Geometry: final body of the model. Coordinates: model frame, mm. Face numbers are marked on the shaded views. A direction names the side the tool comes from. Round coordinates to 2 decimals unless told otherwise and drop trailing zeros. Loops run counter-clockwise (first coordinate to the right, second up) from the corner with the lowest first, then second, coordinate; pieces in that order, holes last. Notation, with made-up numbers: (-34.75, 10) - (-22.75, 10) arc R18 cw to (-22.75, 41) - close; hole circle Ø2 at (59.25, 53.25). An arc over 180 degrees is marked (long way). Return JSON: item names as keys, results as strings. Group by question number.
1. Material intervals for probe 1 along Z at (x, y) = (6.5, 2.5); probe 2 along Z at (x, y) = (8, 4.5); probe 3 along Y at (x, z) = (0.75, 0.95), sorted ascending.
2. Section C-C on z = 0.55. Return loops of the section in (x, y), and give its area (3 significant figures).
3. Section D-D on x = 7.5. Return loops of the section in (y, z).
4. First-contact query: pin 1 Ø0.8 at (x, z) = (4, 0.5) entering from +Y; pin 2 Ø0.8 at (x, z) = (3.5, 0.5) entering from -Y. Flat tips, straight axial feed; report the tip coordinate or a pass-through.
5. Section B-B on x = 5.75. Return loops of the section in (y, z), and give its area (3 significant figures).
6. Set-up query: the marked faces 1, 2 and 3. Return all of +Z, -Z, +X, -X, +Y, -Y with unobstructed straight access to the full face (end or side cutting, diameter ignored); none if empty.
7. Section A-A on y = 0.75. Return loops of the section in (x, z).
from build123d import *

# Parameters (mm, degrees)
SKIZZE1_W                       = 6.912
SKIZZE1_H                       = 3.888
AUFSATZ_LINEAR_AUSTRAGEN1_DEPTH = 1
SKIZZE2_W                       = 10.912
SKIZZE2_H                       = 7.888
AUFSATZ_LINEAR_AUSTRAGEN2_DEPTH = 1
AUFSATZ_LINEAR_AUSTRAGEN3_DEPTH = 0.48
SCHNITT_LINEAR_AUSTRAGEN1_DEPTH = 40.48
SKIZZE7_R                       = 0.1
SCHNITT_LINEAR_AUSTRAGEN2_DEPTH = 0.1
SKIZZE8_R                       = 0.1
SCHNITT_LINEAR_AUSTRAGEN3_DEPTH = 0.1


with BuildPart() as part:
    # Skizze1 → Aufsatz-Linear austragen1 (new body)
    with BuildSketch(Plane.XY):
        with Locations((3.456, 1.944)):
            Rectangle(SKIZZE1_W, SKIZZE1_H)
    extrude(amount=AUFSATZ_LINEAR_AUSTRAGEN1_DEPTH)

    # Skizze2 → Aufsatz-Linear austragen2 (add)
    with BuildSketch(Plane.XY.offset(1)):
        with Locations((3.456, 1.944)):
            Rectangle(SKIZZE2_W, SKIZZE2_H)
    extrude(amount=AUFSATZ_LINEAR_AUSTRAGEN2_DEPTH)

    # Skizze3 → Aufsatz-Linear austragen3 (add)
    with BuildSketch(Plane(origin=(0, 0, 0), x_dir=(-1, 0, 0), z_dir=(0, 0, -1))):
        Polygon((-3.956, 1.944), (-3.456, 2.444), (-2.961061255, 1.949061255), (-3.461061255, 1.449061255), align=None)
    extrude(amount=AUFSATZ_LINEAR_AUSTRAGEN3_DEPTH)

    # Skizze6 → Schnitt-Linear austragen1 (cut)
    with BuildSketch(Plane(origin=(1.006, -1.006, 0), x_dir=(0, 0, -1), z_dir=(0.7071067811865474, -0.7071067811865477, 0))):
        Polygon((0.48, 4.171930009), (0.24, 3.821955466), (0.48, 3.471980924), align=None)
    extrude(amount=-SCHNITT_LINEAR_AUSTRAGEN1_DEPTH, mode=Mode.SUBTRACT)

    # Skizze7 → Schnitt-Linear austragen2 (cut)
    with BuildSketch(Plane(origin=(0.943569205, 0.943569205, -1.945870659), x_dir=(-0.916554971633356, 0.17448706179529924, -0.35983503059071614), z_dir=(0.3999087195525726, 0.3999087195525724, -0.8247096653075213))):
        with Locations(Location((-2.60892888, 1.483064665, 0), (0, 0, 349.02546357))):
            Circle(SKIZZE7_R)
    extrude(amount=-SCHNITT_LINEAR_AUSTRAGEN2_DEPTH, mode=Mode.SUBTRACT)

    # Skizze8 → Schnitt-Linear austragen3 (cut)
    with BuildSketch(Plane(origin=(0.785261084, 0.785261084, 1.619400564), x_dir=(-0.916554971633356, 0.17448706179529927, 0.3598350305907162), z_dir=(-0.3999087195525727, -0.3999087195525724, -0.8247096653075213))):
        with Locations(Location((-3.051649182, 2.019884252, 0), (0, 0, 349.02546357))):
            Circle(SKIZZE8_R)
    extrude(amount=-SCHNITT_LINEAR_AUSTRAGEN3_DEPTH, mode=Mode.SUBTRACT)


solid = part.part
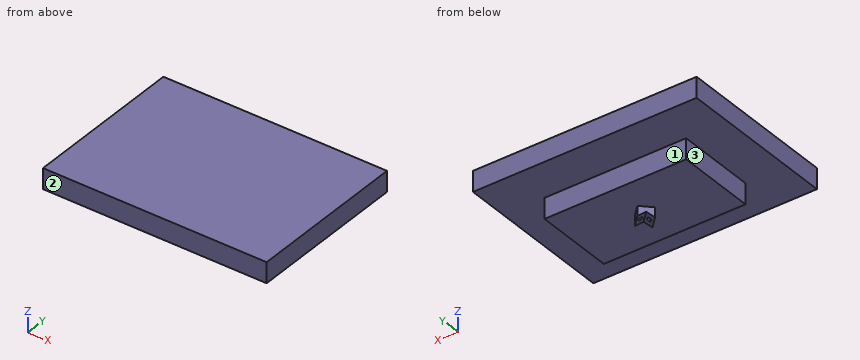
Taken from the geometry:
{
 "1": {"probe 1": "0 to 2", "probe 2": "1 to 2", "probe 3": "0 to 3.89"},
 "2": {"outline": "(0, 0) - (6.91, 0) - (6.91, 3.89) - (0, 3.89) - close", "area": "26.9 mm2"},
 "3": {"outline": "(-2, 1) - (5.89, 1) - (5.89, 2) - (-2, 2) - close"},
 "4": {"pin 1": "y = 3.89", "pin 2": "y = 0"},
 "5": {"outline": "(-2, 1) - (0, 1) - (0, 0) - (3.89, 0) - (3.89, 1) - (5.89, 1) - (5.89, 2) - (-2, 2) - close", "area": "11.8 mm2"},
 "6": {"face 1": "-Z, +X, -X, +Y", "face 2": "+Z, -Z, +X, -X, -Y", "face 3": "-Z, -X, +Y, -Y"},
 "7": {"outline": "(-2, 1) - (0, 1) - (0, 0) - (6.91, 0) - (6.91, 1) - (8.91, 1) - (8.91, 2) - (-2, 2) - close"}
}
